from build123d import *

# Parameters (mm, degrees)
SKETCH1_R                                       = 47.244
SKETCH1_R_2                                     = 34.544
BOSS_EXTRUDE1_DEPTH                             = 8.128
CSK_FOR_M4_FLAT_HEAD_MACHINE_SCREW1_D           = 4.5
CSK_FOR_M4_FLAT_HEAD_MACHINE_SCREW1_CSINK_D     = 9.4
CSK_FOR_M4_FLAT_HEAD_MACHINE_SCREW1_CSINK_ANGLE = 90
CIRPATTERN1_COUNT                               = 4
DRAFT2_ANGLE                                    = 15
SKETCH6_OUTSIDE_W                               = 125.592
SKETCH6_OUTSIDE_H                               = 125.592
SKETCH6_OUTSIDE_R                               = 47.622724369
CUT_EXTRUDE1_DEPTH                              = 69.580417064
FILLET1_R                                       = 6.35
FILLET2_R                                       = 0.79375


with BuildPart() as part:
    # Sketch1 → Boss-Extrude1 (new body)
    with BuildSketch(Plane(origin=(0, 0, 0), x_dir=(1, 0, 0), z_dir=(0, 1, 0))):
        with Locations(Location((0, 0, 0), (0, 0, 270))):
            Circle(SKETCH1_R)
        with Locations(Location((0, 0, 0), (0, 0, 270))):
            Circle(SKETCH1_R_2, mode=Mode.SUBTRACT)
    extrude(amount=BOSS_EXTRUDE1_DEPTH)

    # CSK for M4 Flat Head Machine Screw1 (through all)
    with Locations(Plane(origin=(0, 8.128, -40.894), x_dir=(0, 0, 1), z_dir=(0, 1, 0))):
        with Locations((0, 0)):
            csk_for_m4_flat_head_machine_screw1 = CounterSinkHole(CSK_FOR_M4_FLAT_HEAD_MACHINE_SCREW1_D / 2, CSK_FOR_M4_FLAT_HEAD_MACHINE_SCREW1_CSINK_D / 2, counter_sink_angle=CSK_FOR_M4_FLAT_HEAD_MACHINE_SCREW1_CSINK_ANGLE)

    # CirPattern1: CSK for M4 Flat Head Machine Screw1 ×4 about axis
    cirpattern1_axis = Axis((0, 0, 0), (0, 1, 0))
    for i in range(1, CIRPATTERN1_COUNT):
        add(csk_for_m4_flat_head_machine_screw1.rotate(cirpattern1_axis, i * 360 / CIRPATTERN1_COUNT), mode=Mode.SUBTRACT)

    # Draft2
    draft2_faces = [part.faces().sort_by_distance(p)[0] for p in [
        (0, 4.064, -47.244),
    ]]
    draft(draft2_faces, Plane(origin=(0, 0, 0), x_dir=(0, 0, -1), z_dir=(0, -1, 0)), DRAFT2_ANGLE)

    # Sketch5 → Cut-Revolve1 (revolve, cut)
    with BuildSketch(Plane(origin=(0, 0, 0), x_dir=(0, 0, -1), z_dir=(1, 0, 0)), mode=Mode.PRIVATE) as cut_revolve1_sk:
        Polygon((48.151891036, 8.128), (49.421891036, 8.128), (47.244, 0), (45.974, 0), align=None)
    revolve(cut_revolve1_sk.sketch.rotate(Axis((0, 8.128, 0), (0, -1, 0)), 180), axis=Axis((0, 8.128, 0), (0, -1, 0)), mode=Mode.SUBTRACT)

    # Sketch6 outside → Cut-Extrude1 (cut, through all)
    with BuildSketch(Plane(origin=(0, 8.128, 0), x_dir=(1, 0, 0), z_dir=(0, 1, 0))):
        Rectangle(SKETCH6_OUTSIDE_W, SKETCH6_OUTSIDE_H)
        with Locations(Location((0, 0, 0), (0, 0, 270))):
            Circle(SKETCH6_OUTSIDE_R, mode=Mode.SUBTRACT)
    extrude(amount=-CUT_EXTRUDE1_DEPTH, mode=Mode.SUBTRACT)

    # Fillet1
    fillet1_edges = [part.edges().sort_by_distance(p)[0] for p in [
        (0, 6.153123114, -47.622724369),
    ]]
    fillet(fillet1_edges, radius=FILLET1_R)

    # Fillet2
    fillet2_edges = [part.edges().sort_by_distance(p)[0] for p in [
        (0, 0, -45.974),
        (0, 0, -34.544),
    ]]
    fillet(fillet2_edges, radius=FILLET2_R)


solid = part.part
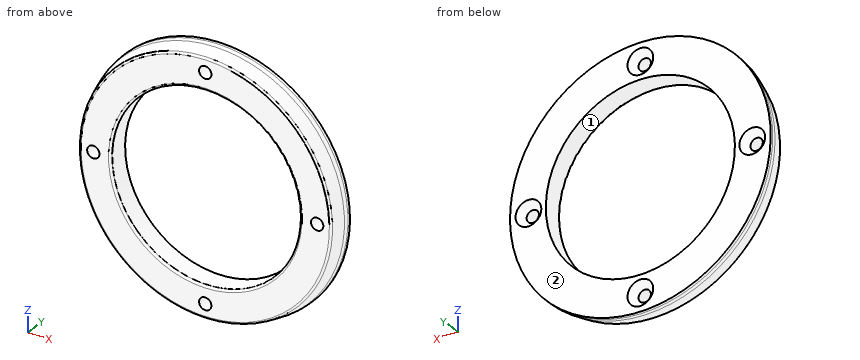
Design review of the part built by this model. Coordinates are the model's own, in mm. Face numbers are marked on the shaded views. Coordinates: 2 decimals unless noted, no trailing zeros. Loops run counter-clockwise (first coordinate to the right, second up) from the corner with the lowest first, then second, coordinate; pieces in that order, holes last. Notation, with made-up numbers: M -40,-30 L -4,-30 A12 cw -4,-18 Z; hole C 82,28 d10. An arc over 180 degrees is marked long. Answer as CSV lines item,"result".
Item 1: The part is to be moulded in two halves that separate along X. For the marked faces 1 and 2, say which applies: pulls with the +X half, pulls with the -X half, needs draft (parallel to the pull), parting line crosses it, or undercut.
Answer list:
face 1,"undercut"
face 2,"needs draft"
Item 2: For P1, Ø3, axis at x = 2, y = 1.5, coming from the -Z side; P2, Ø4, axis at y = 1.5, z = 17.5, coming from the -X side; P3, Ø1.5, axis at x = -21.5, z = 27, coming from the +Y side; P4, Ø7, axis at x = 40.894, z = 0, coming from the +Y side, all flat-tipped, find the tip position at first contact; note any pin that passes through.
Answer list:
P1,"z = -46.74"
P2,"x = -43.91"
P3,"y = 8.13"
P4,"y = 6.93"
Item 3: Add section A-A on z = 0. Count the separate pieces of the cut face and the enclosed holes in it, plus the area to 3 significant figures.
Answer list:
separate pieces,"4"
enclosed holes,"0"
area,"117 mm²"
Item 4: For probe 1 along X at (y, z) = (7, 2.5); probe 2 along Z at (x, y) = (2, 4.5); probe 3 along X at (y, z) = (2.25, 1), list the stretches that pass through material, from the lowest coordinate up.
Answer list:
probe 1,"-47.56 to -43.45, -38.34 to -34.45, 34.45 to 38.34, 43.45 to 47.56"
probe 2,"-47.14 to -41.92, -39.86 to -34.49, 34.49 to 39.86, 41.92 to 47.14"
probe 3,"-46.57 to -42.91, -38.88 to -34.53, 34.53 to 38.88, 42.91 to 46.57"
Item 5: Add section C-C on y = 2. State the section outline as (x, z) points, plus the area to 3 significant figures.
Answer list:
outline,"C 0,0 d93.02; hole C -40.89,0 d4.5; hole C 0,0 d69.09; hole C 0,-40.89 d4.5; hole C 0,40.89 d4.5; hole C 40.89,0 d4.5"
area,"2,980 mm²"
